Verification items for this drawing (mm, ordinates from the low corner). Coordinates: 2 decimals unless noted, no trailing zeros. Write each loop counter-clockwise with the first axis right and the second up, starting at its lowest first coordinate (ties: lowest second). Pieces come first, ordered by that corner, then holes. Notation, with made-up numbers: M 63.5,0.5 L 114.5,0.5 A29 cw 114.5,20.5 Z; hole C -4,-12 d8. An arc over 180 degrees is marked long. Write each question's results on one line, items separated by ' | '.
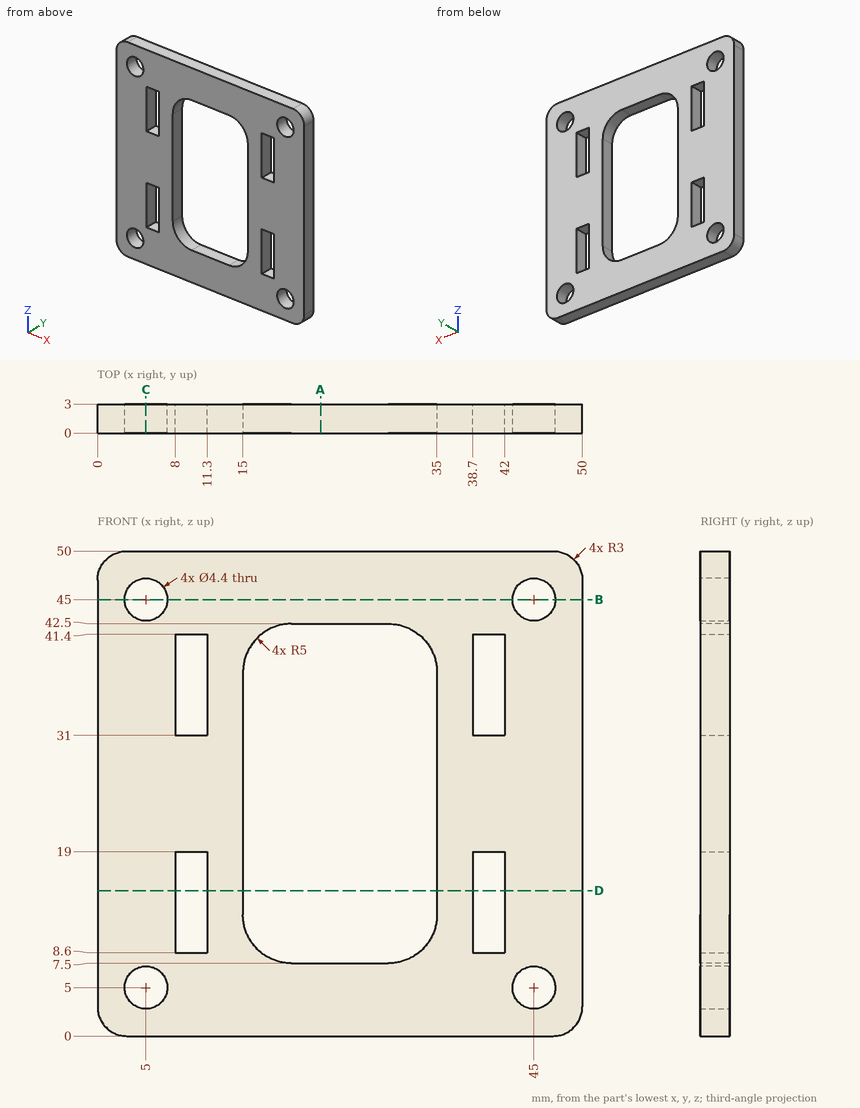
Q1. Sectioned sample at D-D on z = 15. Record the cut outline in (x, y), and give its area (3 significant figures).
Geometry check:
outline: M 0,0 L 8,0 L 8,3 L 0,3 Z; M 11.3,0 L 15,0 L 15,3 L 11.3,3 Z; M 35,0 L 38.7,0 L 38.7,3 L 35,3 Z; M 42,0 L 50,0 L 50,3 L 42,3 Z | area: 70.2 mm2
Q2. Depth check by flat-ended pin: P1, Ø2.5, axis at x = 45, z = 45, coming from the -Y side. Enter the tip coordinate at first touch or a pass-through.
Geometry check:
P1: passes through
Q3. Scan lines: probe 1 along X at (y, z) = (2.8, 45); probe 2 along Z at (x, y) = (9.5, 1.8); probe 3 along Z at (x, y) = (23, 2.35). Record each from-to range of solid material in increasing order.
Geometry check:
probe 1: x = 0 to 2.8, 7.2 to 42.8, 47.2 to 50 | probe 2: z = 0 to 8.6, 19 to 31, 41.4 to 50 | probe 3: z = 0 to 7.5, 42.5 to 50
Q4. Sectioned sample at A-A on x = 23. Record the cut outline in (y, z).
Geometry check:
outline: M 0,0 L 3,0 L 3,7.5 L 0,7.5 Z; M 0,42.5 L 3,42.5 L 3,50 L 0,50 Z
Q5. Sectioned sample at B-B on z = 45. Record the cut outline in (x, y).
Geometry check:
outline: M 0,0 L 2.8,0 L 2.8,3 L 0,3 Z; M 7.2,0 L 42.8,0 L 42.8,3 L 7.2,3 Z; M 47.2,0 L 50,0 L 50,3 L 47.2,3 Z
Q6. Sectioned sample at C-C on x = 5. Record the cut outline in (y, z), and give its area (3 significant figures).
Geometry check:
outline: M 0,0 L 3,0 L 3,2.8 L 0,2.8 Z; M 0,7.2 L 3,7.2 L 3,42.8 L 0,42.8 Z; M 0,47.2 L 3,47.2 L 3,50 L 0,50 Z | area: 124 mm2
